Geometry check sheet. Reference: the model listing, model coordinates, mm. Round coordinates to 2 decimals unless told otherwise and drop trailing zeros. Order: outer loops, then holes, each group sorted by start corner. A loop starts at its lowest first (then second) coordinate and runs counter-clockwise, first axis right, second up.
(1) Cross-section at D-D on z = 6.25. Enter the section's corners in (x, y), and give its area (3 significant figures).
(2) Cross-section at C-C on y = 53. Enter the section's corners in (x, z).
(3) Thickness scan on L1, parallel to Y at x = 0.75, z = 2; L2, parallel to Z at x = -0.5, y = 26; L3, parallel to X at y = 89.5, z = -0.25. Record the ranges inside material, lowest first.
(4) Gauge pin test, flat ends, axial feed: P1, Ø3.5, axis at x = 0.5, y = 4, coming from the -Z side; P2, Ø5, axis at y = 76, z = 5, coming from the +X side; P3, Ø4, axis at y = 55, z = -7.5, coming from the -X side; P4, Ø1.5, axis at x = 6.5, y = 48.5, coming from the +Z side. Record the tip position at first contact, or that the pin passes through.
(5) Cross-section at A-A on x = 0. Enter the section's corners in (y, z), and give its area (3 significant figures).
(6) Cross-section at B-B on z = -1. Enter the section's corners in (x, y).
from build123d import *

# Parameters (mm, degrees)
SKETCH1_R           = 9.5
BOSS_EXTRUDE1_DEPTH = 115
CUT_EXTRUDE1_DEPTH  = 6.6


with BuildPart() as part:
    # Sketch1 → Boss-Extrude1 (new body)
    with BuildSketch(Plane(origin=(0, 0, 0), x_dir=(1, 0, 0), z_dir=(0, 1, 0))):
        Circle(SKETCH1_R)
    extrude(amount=BOSS_EXTRUDE1_DEPTH)

    # Sketch2 → Cut-Extrude1 (cut)
    with BuildSketch(Plane.XZ):
        Polygon((1.610807251, 2.79), (-1.610807251, 2.79), (-3.221614502, 0), (-1.610807251, -2.79), (1.610807251, -2.79), (3.221614502, 0), align=None)
    extrude(amount=-CUT_EXTRUDE1_DEPTH, mode=Mode.SUBTRACT)


solid = part.part
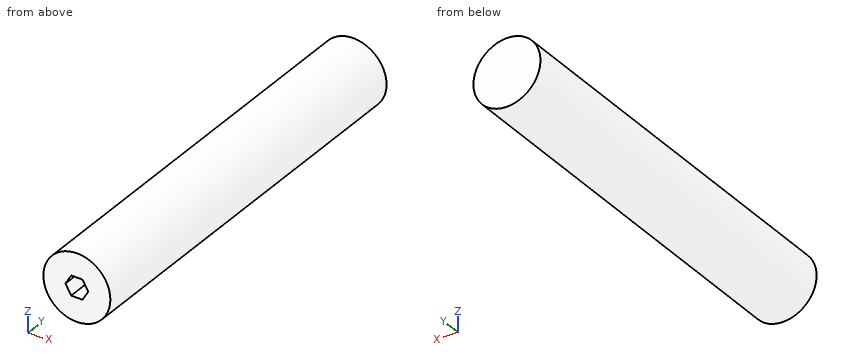
Found:
1. outline: (-7.15, 0) - (7.15, 0) - (7.15, 115) - (-7.15, 115) - close
1. area: 1,650 mm2
2. outline: circle Ø19 at (0, 0)
3. L1: y = 6.6 to 115
3. L2: z = -9.49 to 9.49
3. L3: x = -9.5 to 9.5
4. P1: stops at z = -9.5
4. P2: stops at x = 9.17
4. P3: stops at x = -7.75
4. P4: stops at z = 7.56
5. outline: (0, -9.5) - (115, -9.5) - (115, 9.5) - (0, 9.5) - (0, 2.79) - (6.6, 2.79) - (6.6, -2.79) - (0, -2.79) - close
5. area: 2,150 mm2
6. outline: (-9.45, 0) - (-2.64, 0) - (-2.64, 6.6) - (2.64, 6.6) - (2.64, 0) - (9.45, 0) - (9.45, 115) - (-9.45, 115) - close
